Can you work these out from the model? Positions are in its coordinate system, mm. A direction names the side the tool comes from. Round coordinates to 2 decimals unless told otherwise and drop trailing zeros. Order: outer loops, then holes, each group sorted by start corner. A loop starts at its lowest first (then second) coordinate and runs counter-clockwise, first axis right, second up.
Q1. Will these pins go through, and if not, where does the flat tip stop? P1, Ø4.5, axis at x = 17, z = 0, coming from the +Y side; P2, Ø3, axis at x = 4.5, z = 5.5, coming from the -Y side; P3, Ø6.5, axis at x = 0, y = 31.01, coming from the -Z side; P4, Ø4.5, axis at y = 24, z = -0.5, coming from the -X side.
Q2. If we section it at C-C (z = 5.75): Please give me the cut outline in (x, y), plus the area to 3 significant figures.
Q3. We'd pull the mould along X, two halves only. Please class faces 4 (the face through (22.699, -2.715, 0.105)), 5 (the face through (-22.699, 11.715, 0.105)), 6 (the face through (0, 0, 0)), 7 (the face through (3, 42, 0)): pulls with the +X half, pulls with the -X half, needs draft (parallel to the pull), parting line crosses it, or undercut.
Q4. For faces 1 (the face through (0.998, 39, 2)), 2 (the face through (-20.301, -2.715, -0.105)), 3 (the face through (0, 15, -7.5)), which set-ups out of +Z, -Z, +X, -X, +Y, -Y let a thin tool reach every point of the face, with its end or its side?
Q5. If we section it at D-D (y = 9.5): Please give me the cut outline in (x, z), plus the area to 3 significant figures.
Q6. If we section it at A-A (y = 38): Please give me the cut outline in (x, z), plus the area to 3 significant figures.
Q7. If I drill on line 1 (Z direction, x = 17, y = 9.25); line 2 (X direction, y = 38, z = -6.25); line 3 (X direction, y = 14.5, z = -5.25), over which ranges is the centre line in solid material (lowest first)?
Q8. If we section it at B-B (x = 17): Please give me the cut outline in (y, z).
from build123d import *

# Parameters (mm, degrees)
SKETCH002_R  = 2
PAD002_DEPTH = 17.5
SKETCH001_R  = 2
PAD001_DEPTH = 20
PAD_DEPTH    = 7.5
FILLET_R     = 1


with BuildPart() as pad002:
    # Sketch002 → Pad002 (new body, symmetric)
    with BuildSketch(Plane.YZ):
        with Locations((38, 0)):
            Circle(SKETCH002_R)
    extrude(amount=PAD002_DEPTH, both=True)


with BuildPart() as pad001:
    # Sketch001 → Pad001 (new body, symmetric)
    with BuildSketch(Plane.XZ):
        with Locations((-17, 0)):
            Circle(SKETCH001_R)
        with Locations((17, 0)):
            Circle(SKETCH001_R)
    extrude(amount=PAD001_DEPTH, both=True)


with BuildPart() as fillet_body:
    # Sketch → Pad (new body, symmetric)
    with BuildSketch(Plane.XY):
        with BuildLine():
            Line((0, 0), (20, 0))
            Line((20, 0), (20, -3))
            Line((20, -3), (23, -3))
            Line((23, -3), (23, 12))
            Line((23, 12), (7, 12))
            Line((7, 12), (7, 42))
            Line((0.998309, 42), (7, 42))
            Line((0.998309, 34.901094), (0.998309, 42))
            ThreePointArc((0, 35.026635), (-0.499717, 27.020731), (0.998309, 34.901094))
            Line((0, 42), (0, 35.026635))
            Line((-7, 42), (0, 42))
            Line((-7, 42), (-7, 12))
            Line((-7, 12), (-23, 12))
            Line((-23, -3), (-23, 12))
            Line((-20, -3), (-23, -3))
            Line((-20, 0), (-20, -3))
            Line((0, 0), (-20, 0))
        make_face()
    extrude(amount=PAD_DEPTH, both=True)

    # Cut: cut Pad001
    add(pad001.part, mode=Mode.SUBTRACT)

    # Cut001: cut Pad002
    add(pad002.part, mode=Mode.SUBTRACT)

    # Fillet
    fillet_edges = [fillet_body.edges().sort_by_distance(p)[0] for p in [
        (23, -3, 0),
        (20, -3, 0),
        (-20, -3, 0),
        (-23, -3, 0),
        (23, 12, 0),
        (7, 42, 0),
        (-0.499717, 27.020731, 7.5),
        (-23, 12, 0),
        (-7, 42, 0),
        (-0.499717, 27.020731, -7.5),
    ]]
    fillet(fillet_edges, radius=FILLET_R)


solid = fillet_body.part
Solution:
1. P1: stops at y = 12
1. P2: stops at y = 0
1. P3: passes through
1. P4: stops at x = -7
2. outline: (-23, -2) arc R1 ccw to (-22, -3) - (-21, -3) arc R1 ccw to (-20, -2) - (-20, 0) - (20, 0) - (20, -2) arc R1 ccw to (21, -3) - (22, -3) arc R1 ccw to (23, -2) - (23, 11) arc R1 ccw to (22, 12) - (7, 12) - (7, 41) arc R1 ccw to (6, 42) - (1, 42) - (1, 34.9) arc R4.02 cw (long way) to (0, 35.03) - (0, 42) - (-6, 42) arc R1 ccw to (-7, 41) - (-7, 12) - (-22, 12) arc R1 ccw to (-23, 11) - close
2. area: 931 mm2
3. face 4: pulls with the +X half
3. face 5: pulls with the -X half
3. face 6: undercut
3. face 7: needs draft
4. face 1: +Z, -Z, +Y
4. face 2: +Z, -Z, -Y
4. face 3: -Z, +X, -X, +Y, -Y
5. outline: (-23, -7.5) - (23, -7.5) - (23, 7.5) - (-23, 7.5) - close; hole circle Ø4 at (-17, 0); hole circle Ø4 at (17, 0)
5. area: 665 mm2
6. outline: (-7, -7.5) - (0, -7.5) - (0, -2) - (-7, -2) - close; (-7, 2) - (0, 2) - (0, 7.5) - (-7, 7.5) - close; (1, -7.5) - (7, -7.5) - (7, -2) - (1, -2) - close; (1, 2) - (7, 2) - (7, 7.5) - (1, 7.5) - close
6. area: 143 mm2
7. line 1: z = -7.5 to -2, 2 to 7.5
7. line 2: x = -7 to 0, 1 to 7
7. line 3: x = -7 to 7
8. outline: (0, -7.5) - (12, -7.5) - (12, -2) - (0, -2) - close; (0, 2) - (12, 2) - (12, 7.5) - (0, 7.5) - close
